from build123d import *

# Parameters (mm, degrees)
SKETCH_1_W          = 22
SKETCH_1_H          = 12
EXTRUDE_1_DEPTH     = 22
EXTRUDE_2_DEPTH     = 5
SKETCH_4_R          = 2
EXTRUDE_3_DEPTH     = 3
SKETCH_5_W          = 5
SKETCH_5_H          = 2
EXTRUDE_4_DEPTH     = 12
SKETCH_6_W          = 3
SKETCH_6_H          = 1.5
EXTRUDE_5_DEPTH     = 3
CUT_EXTRUDE_1_DEPTH = 3


with BuildPart() as part:
    # 草图1 → 凸台-拉伸1 (new body)
    with BuildSketch(Plane(origin=(0, 0, 0), x_dir=(1, 0, 0), z_dir=(0, 1, 0))):
        Rectangle(SKETCH_1_W, SKETCH_1_H)
    extrude(amount=EXTRUDE_1_DEPTH)

    # 草图3 → 凸台-拉伸2 (add)
    with BuildSketch(Plane(origin=(0, 22, 0), x_dir=(1, 0, 0), z_dir=(0, 1, 0))):
        with BuildLine():
            ThreePointArc((0.479166667, 2.445144707), (-11, 0), (0.479166667, -2.445144707))
            ThreePointArc((0.479166667, -2.445144707), (3.5, 0), (0.479166667, 2.445144707))
        make_face()
    extrude(amount=EXTRUDE_2_DEPTH)

    # 草图4 → 凸台-拉伸3 (add)
    with BuildSketch(Plane(origin=(0, 27, 0), x_dir=(1, 0, 0), z_dir=(0, 1, 0))):
        with Locations((-5, 0)):
            Circle(SKETCH_4_R)
    extrude(amount=EXTRUDE_3_DEPTH)

    # 草图5 → 凸台-拉伸4 (add)
    with BuildSketch(Plane.XY.offset(6)):
        with Locations((-13.5, 17)):
            Rectangle(SKETCH_5_W, SKETCH_5_H)
        with Locations((13.5, 17)):
            Rectangle(SKETCH_5_W, SKETCH_5_H)
    extrude(amount=-EXTRUDE_4_DEPTH)

    # 草图6 → 凸台-拉伸5 (add)
    with BuildSketch(Plane.ZY.offset(11)):
        with Locations((0, 5.75)):
            Rectangle(SKETCH_6_W, SKETCH_6_H)
    extrude(amount=EXTRUDE_5_DEPTH)

    # 草图7 → 切除-拉伸1 (cut)
    with BuildSketch(Plane(origin=(0, 18, 0), x_dir=(1, 0, 0), z_dir=(0, 1, 0))):
        with BuildLine():
            Line((-16, -0.495646194), (-14.868524525, -0.495646194))
            ThreePointArc((-14.868524525, -0.495646194), (-13.000012637, -0.005027364), (-14.863497098, 0.504353806))
            Line((-14.863497098, 0.504353806), (-16, 0.504353806))
            Line((-16, 0.504353806), (-16, -0.495646194))
        make_face()
        with BuildLine():
            Line((14.866025404, -0.5), (16, -0.5))
            Line((16, -0.5), (16, 0.5))
            Line((16, 0.5), (14.866025404, 0.5))
            ThreePointArc((14.866025404, 0.5), (13, 0), (14.866025404, -0.5))
        make_face()
    extrude(amount=-CUT_EXTRUDE_1_DEPTH, mode=Mode.SUBTRACT)


solid = part.part
Could you check a few things on this model? Use its own coordinates, in mm. A direction names the side the tool comes from. Coordinates: 2 decimals unless noted, no trailing zeros. Order: outer loops, then holes, each group sorted by start corner. A loop starts at its lowest first (then second) coordinate and runs counter-clockwise, first axis right, second up. Notation, with made-up numbers: (30.5, -26.5) -> (56.5, -26.5) arc R28 cw to (56.5, -8.5) -> close; hole circle Ø1 at (36.25, -19.75). An arc over 180 degrees is marked (long way). One line per item, written item: value. Start each with the question number.
1) Imagine slicing it at B-B on x = 1. List the corners of the cut face in (y, z) for me.
2) We'd pull the mould along Z, two halves only. Please class faces 6 (the flat face through (-12, 6, -1.5)), 7 (the flat face through (-5, 30, 0)), 8 (the flat face through (-15.4, 17, -0.504)): +Z half, -Z half, draft (parallel to the pull), parting line (faces both ways), or undercut.
3) Imagine slicing it at D-D on y = 18.75. List the corners of the cut face in (x, z) for me.
4) If I drill on L1, parallel to Z at x = -14, y = 17.1; L2, parallel to Y at x = 3, z = -1.75; L3, parallel to X at y = 21.25, z = 1, over which ranges is the centre line in solid material (lowest first)? Write a range as [from, to].
5) Which directions (+Z, -Z, +X, -X, +Y, -Y) give clear straight access to the entire face, cutting with the end or side of a thin tool? Please do faces 1 (the cylindrical face through (-13, 17, 0)), 2 (the flat face through (15.4, 17, 0.5)), 3 (the flat face through (-14, 6, 0)), 4 (the flat face through (11, 8, 0)), 5 (the flat face through (-11, 20, 0)).
6) Imagine slicing it at A-A on x = 14. List the corners of the cut face in (y, z) for me, plus the area to 3 significant figures.
7) Imagine slicing it at C-C on z = 3.5. List the corners of the cut face in (x, y) for me.
8) I'm going to push flat-ended pins straight in: pin 1 (1.6 mm diameter, centred on x = -12, y = 5.5, fed in from -Z); pin 2 (4 mm diameter, centred on x = -13.5, z = 2.5, fed in from -Y); pin 3 (5 mm diameter, centred on y = 22, z = 0.5, fed in from +X). Where does each tip first touch, or does it pass through?
Answer list:
1. outline: (0, -6) -> (22, -6) -> (22, -2.5) -> (27, -2.5) -> (27, 2.5) -> (22, 2.5) -> (22, 6) -> (0, 6) -> close
2. face 6: -Z half
2. face 7: draft
2. face 8: undercut
3. outline: (-11, -6) -> (11, -6) -> (11, 6) -> (-11, 6) -> close
4. L1: z = [-6, -1], [1, 6]
4. L2: y = [0, 22]
4. L3: x = [-11, 11]
5. face 1: +Y
5. face 2: +X, +Y, -Y
5. face 3: +Z, -Z, -X, -Y
5. face 4: +Z, -Z, +X, -Y
5. face 5: +Z, -Z, -X, +Y
6. outline: (16, -6) -> (18, -6) -> (18, -1) -> (16, -1) -> close; (16, 1) -> (18, 1) -> (18, 6) -> (16, 6) -> close
6. area: 20.0 mm2
7. outline: (-16, 16) -> (-11, 16) -> (-11, 0) -> (11, 0) -> (11, 16) -> (16, 16) -> (16, 18) -> (11, 18) -> (11, 22) -> (-0.13, 22) -> (-0.13, 27) -> (-9.87, 27) -> (-9.87, 22) -> (-11, 22) -> (-11, 18) -> (-16, 18) -> close
8. pin 1: stops at z = -1.5
8. pin 2: stops at y = 5
8. pin 3: stops at x = 11
